Read the model definition and answer for the solid it produces. Units are mm, in the model's axes. A direction names the side the tool comes from. Coordinates: 2 decimals unless noted, no trailing zeros. Write each loop counter-clockwise with the first axis right and the second up, starting at its lowest first coordinate (ties: lowest second). Pieces come first, ordered by that corner, then holes.
(1) Section B-B on x = 22 is taken. Write down the section's boundary in (y, z), then the cut area to 3 significant figures.
(2) The mould has two halves that part along Y. Classify faces 1 (the flat face through (-1, -20, 10)), 2 (the cylindrical face through (-20.634, -0.493, 21.083)), 3 (the flat face through (-12, 0, -12)): +Y half, -Y half, draft (parallel to the pull), parting line (faces both ways), or undercut.
(3) Section C-C on y = -17.5 is taken. Write down the section's boundary in (x, z).
(4) Find the intervals of material crossed by probe 1 along Z at (x, y) = (0, -0.65); probe 2 along Z at (x, y) = (-18, -7.25), in increasing order.
(5) Section A-A on y = -4.5 is taken. Write down the section's boundary in (x, z), then the cut area to 3 significant figures.
(6) Which of the six approach directions +Z, -Z, +X, -X, +Y, -Y give full straight-line access (tool end or side, diameter ignored) to faces 4 (the flat face through (-12, 0, 12)), 5 (the cylindrical face through (20.634, -0.493, -21.083))?
(7) Given pin 1 (6 mm diameter, centred on x = 20, y = -4.5, fed in from -Z); pin 2 (5 mm diameter, centred on y = -5.5, z = -31.5, fed in from -X); pin 3 (3 mm diameter, centred on y = -9.5, z = -1, fed in from -X), each flat-ended and moving along its own axis, determine where each tip first touches the part or whether it passes through.
(8) Section D-D on x = 36.5 is taken. Write down the section's boundary in (y, z).
from build123d import *

# Parameters (mm, degrees)
SKETCH2_R                                = 50
BOSS_EXTRUDE2_DEPTH                      = 20
SKETCH1_R                                = 30
CUT_EXTRUDE1_DEPTH                       = 1
F_60_0_04_DIAMETER_HOLE1_D               = 1.016
F_60_0_04_DIAMETER_HOLE1_DEPTH           = 10
F_60_0_04_DIAMETER_HOLE1_TIP             = 0.305237194
F_60_0_04_DIAMETER_HOLE1_ON_FACE_2_D     = 1.016
F_60_0_04_DIAMETER_HOLE1_ON_FACE_2_DEPTH = 10
F_60_0_04_DIAMETER_HOLE1_ON_FACE_2_TIP   = 0.305237194
F_2_0_221_DIAMETER_HOLE1_D               = 5.6134
F_2_0_221_DIAMETER_HOLE1_DEPTH           = 55
F_2_0_221_DIAMETER_HOLE1_TIP             = 1.686435499


with BuildPart() as part:
    # Sketch2 → Boss-Extrude2 (new body)
    with BuildSketch(Plane(origin=(0, 0, 0), x_dir=(1, 0, 0), z_dir=(0, 1, 0))):
        Circle(SKETCH2_R)
    extrude(amount=-BOSS_EXTRUDE2_DEPTH)

    # Sketch1 → Cut-Extrude1 (cut)
    with BuildSketch(Plane(origin=(0, 0, 0), x_dir=(1, 0, 0), z_dir=(0, 1, 0))):
        Circle(SKETCH1_R)
        with BuildLine():
            Line((-0.5, -0.5), (-0.5, -29.495762408))
            ThreePointArc((-0.5, -29.495762408), (-20.859650045, -20.859650045), (-29.495762408, -0.5))
            Line((-29.495762408, -0.5), (-0.5, -0.5))
        make_face(mode=Mode.SUBTRACT)
        with BuildLine():
            ThreePointArc((29.495762408, -0.5), (20.859650045, -20.859650045), (0.5, -29.495762408))
            Line((0.5, -29.495762408), (0.5, -0.5))
            Line((0.5, -0.5), (29.495762408, -0.5))
        make_face(mode=Mode.SUBTRACT)
        with BuildLine():
            Line((-0.5, 29.495762408), (-0.5, 0.5))
            Line((-0.5, 0.5), (-29.495762408, 0.5))
            ThreePointArc((-29.495762408, 0.5), (-20.859650045, 20.859650045), (-0.5, 29.495762408))
        make_face(mode=Mode.SUBTRACT)
        with BuildLine():
            Line((29.495762408, 0.5), (0.5, 0.5))
            Line((0.5, 0.5), (0.5, 29.495762408))
            ThreePointArc((0.5, 29.495762408), (20.859650045, 20.859650045), (29.495762408, 0.5))
        make_face(mode=Mode.SUBTRACT)
    extrude(amount=-CUT_EXTRUDE1_DEPTH, mode=Mode.SUBTRACT)

    # #60 (0.04) Diameter Hole1
    with Locations(Plane(origin=(9.64e-06, -1, -4.709e-06), x_dir=(0, 0, 1), z_dir=(0, 1, 0))):
        with Locations((0, 0)):
            Hole(F_60_0_04_DIAMETER_HOLE1_D / 2, depth=F_60_0_04_DIAMETER_HOLE1_DEPTH)
            with Locations((0, 0, -(F_60_0_04_DIAMETER_HOLE1_DEPTH + F_60_0_04_DIAMETER_HOLE1_TIP / 2))):  # 118° drill point
                Cone(0, F_60_0_04_DIAMETER_HOLE1_D / 2, F_60_0_04_DIAMETER_HOLE1_TIP, mode=Mode.SUBTRACT)

    # #60 (0.04) Diameter Hole1 on face 2
    with Locations(Plane.ZX):
        with Locations((0, 0)):
            Hole(F_60_0_04_DIAMETER_HOLE1_ON_FACE_2_D / 2, depth=F_60_0_04_DIAMETER_HOLE1_ON_FACE_2_DEPTH)
            with Locations((0, 0, -(F_60_0_04_DIAMETER_HOLE1_ON_FACE_2_DEPTH + F_60_0_04_DIAMETER_HOLE1_ON_FACE_2_TIP / 2))):  # 118° drill point
                Cone(0, F_60_0_04_DIAMETER_HOLE1_ON_FACE_2_D / 2, F_60_0_04_DIAMETER_HOLE1_ON_FACE_2_TIP, mode=Mode.SUBTRACT)

    # #2 (0.221) Diameter Hole1
    with Locations(Plane(origin=(-50, -9.832744337, 1.0253e-05), x_dir=(-2.05e-07, 0, -1), z_dir=(-1, 0, 2.05e-07))):
        with Locations((0, 0), (1.0253e-05, -1.9e-08)):
            Hole(F_2_0_221_DIAMETER_HOLE1_D / 2, depth=F_2_0_221_DIAMETER_HOLE1_DEPTH)
            with Locations((0, 0, -(F_2_0_221_DIAMETER_HOLE1_DEPTH + F_2_0_221_DIAMETER_HOLE1_TIP / 2))):  # 118° drill point
                Cone(0, F_2_0_221_DIAMETER_HOLE1_D / 2, F_2_0_221_DIAMETER_HOLE1_TIP, mode=Mode.SUBTRACT)

    # Sketch9 → Cut-Revolve1 (revolve, cut)
    with BuildSketch(Plane(origin=(0, -20, 0), x_dir=(-1, 0, 0), z_dir=(0, -1, 0))):
        with BuildLine():
            Line((-5, 0), (5, 0))
            ThreePointArc((5, 0), (0, 5), (-5, 0))
        make_face()
    revolve(axis=Axis((5, -20, 0), (-1, 0, 0)), mode=Mode.SUBTRACT)


solid = part.part
Response:
1. outline: (-20, -44.9) - (0, -44.9) - (0, -20.4) - (-1, -20.4) - (-1, -19.65) - (0, -19.65) - (0, -0.5) - (-1, -0.5) - (-1, 0.5) - (0, 0.5) - (0, 19.65) - (-1, 19.65) - (-1, 20.4) - (0, 20.4) - (0, 44.9) - (-20, 44.9) - close
1. area: 1,790 mm2
2. face 1: -Y half
2. face 2: draft
2. face 3: +Y half
3. outline: circle Ø100 at (0, 0); hole circle Ø8.66 at (0, 0)
4. probe 1: z = -50 to -30, 30 to 50
4. probe 2: z = -46.65 to -1.1, 1.1 to 46.65
5. outline: circle Ø100 at (0, 0); hole (-0.22, -0.46) arc R0.51 ccw to (0.22, 0.46) arc R0.51 ccw to start
5. area: 7,850 mm2
6. face 4: +Z, -Z, +X, -X, +Y
6. face 5: +Y
7. pin 1: stops at z = -47.02
7. pin 2: stops at x = -40.73
7. pin 3: stops at x = 5.15
8. outline: (-20, -34.17) - (0, -34.17) - (0, 34.17) - (-20, 34.17) - close
